The listing builds one solid part. Answer for the finished solid, in the listing's coordinates (mm). Give positions to 0.01 mm unless a question says otherwise; leave off trailing zeros. Write each loop counter-clockwise with the first axis right and the second up, starting at its lowest first coordinate (ties: lowest second). Pieces come first, ordered by that corner, then holes. Notation, with made-up numbers: (53.25, 71) -> (89.25, 71) arc R12 ccw to (89.25, 80) -> close; hole circle Ø4 at (31, 78). An arc over 180 degrees is marked (long way). One line per question, with ' | ' between items.
from build123d import *

# Parameters (mm, degrees)
SKETCH1_R           = 1
BOSS_EXTRUDE1_DEPTH = 1


with BuildPart() as part:
    # Sketch1 → Boss-Extrude1 (new body)
    with BuildSketch(Plane.XY):
        with BuildLine():
            Line((-0.021163243, 2.499910422), (-14.978836757, 2.499910422))
            ThreePointArc((-14.978836757, 2.499910422), (-17.499977605, 0.010581716), (-15, -2.5))
            Line((-15, -2.5), (0, -2.5))
            ThreePointArc((0, -2.5), (2.499977605, -0.010581716), (0.021163243, 2.499910422))
            Line((0.021163243, 2.499910422), (-0.021163243, 2.499910422))
        make_face()
        with Locations((-15, 0)):
            Circle(SKETCH1_R, mode=Mode.SUBTRACT)
        Circle(SKETCH1_R, mode=Mode.SUBTRACT)
    extrude(amount=BOSS_EXTRUDE1_DEPTH)


solid = part.part
Item 1: Determine the mould class of faces 1 (the face through (2.5, -0.1, 0.5)), 2 (the face through (-8, 0, 1)), 3 (the face through (-14.046, 0.3, 0.493)) for opening direction Y: pulls with the +Y half, pulls with the -Y half, needs draft (parallel to the pull), parting line crosses it, or undercut.
Answers below:
face 1: parting line crosses it | face 2: needs draft | face 3: undercut
Item 2: Find section B-B (x = -15.5). Write down the section's boundary in (y, z).
Answers below:
outline: (-2.45, 0) -> (-0.87, 0) -> (-0.87, 1) -> (-2.45, 1) -> close; (0.87, 0) -> (2.45, 0) -> (2.45, 1) -> (0.87, 1) -> close
Item 3: Find section A-A (y = 0). Write down the section's boundary in (x, z), then the cut area to 3 significant figures.
Answers below:
outline: (-17.5, 0) -> (-16, 0) -> (-16, 1) -> (-17.5, 1) -> close; (-14, 0) -> (-1, 0) -> (-1, 1) -> (-14, 1) -> close; (1, 0) -> (2.5, 0) -> (2.5, 1) -> (1, 1) -> close | area: 16.0 mm²
Item 4: Consider line 1 (X direction, y = -0.05, z = 0.6); line 2 (Y direction, x = 0, z = 0.75); line 3 (X direction, y = -2.2, z = 0.6). Determine where each line is inside the solid, lowest interval first. Write a range as [from, to].
Answers below:
line 1: [-17.5, -16], [-14, -1], [1, 2.5] | line 2: [-2.5, -1], [1, 2.5] | line 3: [-16.19, 1.19]
Item 5: Find section C-C (z = 0.7). Write down the section's boundary in (x, y).
Answers below:
outline: (-15, -2.5) -> (0, -2.5) arc R2.5 ccw to (0.02, 2.5) -> (-14.98, 2.5) arc R2.5 ccw (long way) to start; hole circle Ø2 at (-15, 0); hole circle Ø2 at (0, 0)
